Can you work these out from the model? Positions are in its coordinate system, mm. A direction names the side the tool comes from. Coordinates: 2 decimals unless noted, no trailing zeros. Write each loop counter-clockwise with the first axis right and the second up, starting at its lowest first coordinate (ties: lowest second). Pieces come first, ordered by that corner, then holes. Notation, with made-up numbers: (23.5, 36) - (68.5, 36) arc R28 cw to (68.5, 66) - close; hole circle Ø11 at (30, -8). An arc over 180 degrees is marked (long way). One line per question, with ' | ' between items. Start each with the question number.
from build123d import *

# Parameters (mm, degrees)
SKETCH1_R           = 4.7625
BOSS_EXTRUDE1_DEPTH = 6.35
FILLET1_R           = 6.35
FILLET2_R           = 9.525
SKETCH3_R           = 3.175
CUT_EXTRUDE2_DEPTH  = 49.046468393


with BuildPart() as part:
    # Sketch1 → Boss-Extrude1 (new, symmetric)
    with BuildSketch(Plane.XY):
        Polygon((-9.525, 22.225), (-9.525, -9.525), (9.525, -9.525), (9.525, 22.225), (28.575, 22.225), (28.575, 28.575), (-28.575, 28.575), (-28.575, 22.225), align=None)
        Circle(SKETCH1_R, mode=Mode.SUBTRACT)
    extrude(amount=BOSS_EXTRUDE1_DEPTH, both=True)

    # Fillet1
    fillet1_edges = [part.edges().sort_by_distance(p)[0] for p in [
        (9.525, 22.225, 0),
        (-9.525, 22.225, 0),
    ]]
    fillet(fillet1_edges, radius=FILLET1_R)

    # Fillet2
    fillet2_edges = [part.edges().sort_by_distance(p)[0] for p in [
        (9.525, -9.525, 0),
        (-9.525, -9.525, 0),
    ]]
    fillet(fillet2_edges, radius=FILLET2_R - 0.0001)  # a hair under: the kernel refuses the full size

    # Sketch3 → Cut-Extrude2 (cut, through all)
    with BuildSketch(Plane(origin=(0, 28.575, 0), x_dir=(1, 0, 0), z_dir=(0, 1, 0))):
        with Locations(Location((-22.225, 0, 0), (0, 0, 180))):
            Circle(SKETCH3_R)
        with Locations(Location((22.225, 0, 0), (0, 0, 180))):
            Circle(SKETCH3_R)
    extrude(amount=-CUT_EXTRUDE2_DEPTH, mode=Mode.SUBTRACT)


solid = part.part
(1) If I drill on probe 1 along Y at (x, z) = (0, 0.5) (1 decimal); probe 2 along Y at (x, z) = (-17, -4.75) (3 decimals); probe 3 along X at (y, z) = (24.5, 1) (3 decimals), over which ranges is the centre line in solid material (lowest first)?
(2) If we mould it in two halves opening along Y, with no side actions, what happens to faces 4 (the face through (-6.81, -6.66, 0.09)), 5 (the face through (28.575, 25, 0)), 6 (the face through (-3.78, -2.9, -0.09))? For each: +Y half, -Y half, draft (parallel to the pull), parting line (faces both ways), or undercut.
(3) If we section it at B-B on y = 24: List the corners of the cut face in (x, z) for me (3 decimals).
(4) I'm going to push flat-ended pins straight in: pin 1 (4 mm diameter, centred on x = 23.5, z = 2.5, fed in from -Y) (3 decimals); pin 2 (4 mm diameter, centred on y = 10, z = -2.5, fed in from -X) (3 decimals). Where does each tip first touch, or does it pass through?
(5) Which directions (+Z, -Z, +X, -X, +Y, -Y) give clear straight access to the entire face, cutting with the end or side of a thin tool? Please do faces 1 (the face through (9.525, 8, 0)), 2 (the face through (-9.525, 8, 0)), 3 (the face through (19.197, 25.444, 0.954)).
(6) If we section it at A-A on z = 0: Give the number of separate pieces and of enclosed holes in the cut face, plus the area to 3 significant figures.
(7) If we section it at C-C on x = 20.5: List the corners of the cut face in (y, z) for me (3 decimals).
Values:
1) probe 1: -9.5 to -4.8, 4.8 to 28.6 | probe 2: 22.225 to 28.575 | probe 3: -28.575 to -25.238, -19.212 to 19.212, 25.238 to 28.575
2) face 4: -Y half | face 5: draft | face 6: undercut
3) outline: (-28.575, -6.35) - (28.575, -6.35) - (28.575, 6.35) - (-28.575, 6.35) - close; hole circle Ø6.35 at (-22.225, 0); hole circle Ø6.35 at (22.225, 0)
4) pin 1: y = 22.225 | pin 2: x = -9.525
5) face 1: +Z, -Z, +X, -Y | face 2: +Z, -Z, -X, -Y | face 3: +Y, -Y
6) separate pieces: 3 | enclosed holes: 1 | area: 794 mm2
7) outline: (22.225, -6.35) - (28.575, -6.35) - (28.575, -2.666) - (22.225, -2.666) - close; (22.225, 2.666) - (28.575, 2.666) - (28.575, 6.35) - (22.225, 6.35) - close
